Part model, mm, in its own coordinate system. Round coordinates to 2 decimals unless told otherwise and drop trailing zeros. Return JSON: item names as keys, results as strings. Group by question number.
(1) Mould opens along Y. For faces 1 (the flat face through (6, -10, -113)), 2 (the cylindrical face through (-0.631, 2.003, -113.39)), 3 (the flat face through (6, 10, -113)) say: +Y half, -Y half, draft (parallel to the pull), parting line (faces both ways), or undercut.
(2) Drill centre lines: L1, parallel to Y at x = 0, z = -156; L2, parallel to Y at x = -7.25, z = -218.5. Where is each one in solid material? Low to high. Write a range as from..to.
(3) Drop flat-ended pins along their axis: pin 1 Ø2 at (x, z) = (9.5, -172) entering from +Y; pin 2 Ø0.7 at (y, z) = (-2.5, -154) entering from +X; pin 3 Ø0.5 at (x, z) = (-2.5, -84) entering from +Y; pin 4 Ø1.5 at (x, y) = (-0.5, -6) entering from +Z. Give the stop position or say it passes through.
Autodesk Inventor part; units mm, degrees
ref_plane "C1_XY" through (0, 0, 0) normal (0, 0, 1) x (1, 0, 0)
ref_plane "C1_YZ" through (0, 0, 0) normal (1, 0, 0) x (0, 1, 0)
ref_plane "C1_ZX" through (0, 0, 0) normal (0, 1, 0) x (0, 0, 1)
sketch "Sketch_75" plane through (0, 0, 0) normal (0, 0, 1) x (1, 0, 0)
  line L0 (-10, 3) -> (-8, 3)
  line L1 (-8, 3) -> (-8, 6)
  line L2 (-8, 6) -> (-7.0607, 6)
  line L3 (-7.0607, 6) -> (-4, 2.9393)
  line L4 (-4, 2.9393) -> (-4, 0.6536)
  arc A0 (-4, 0.6536) -> (-3.933, 0.4036) centre (-3.5, 0.6536) ccw
  line L5 (-3.933, 0.4036) -> (-3.7, 0)
  line L6 (-3.7, 0) -> (-3.933, -0.4036)
  arc A1 (-3.933, -0.4036) -> (-3.933, -0.9036) centre (-3.5, -0.6536) ccw
  line L7 (-3.933, -0.9036) -> (-3.751, -1.2189)
  line L8 (-3.751, -1.2189) -> (-4, -2.5)
  line L9 (-4, -2.5) -> (-4, -2.9393)
  line L10 (-4, -2.9393) -> (-7.0607, -6)
  line L11 (-7.0607, -6) -> (-8, -6)
  line L12 (-8, -6) -> (-8, -3)
  line L13 (-8, -3) -> (-10, -3)
  line L14 (-10, -3) -> (-10, -9)
  arc A2 (-10, -9) -> (-9, -10) centre (-9, -9) ccw
  line L15 (-9, -10) -> (-3, -10)
  line L16 (-3, -10) -> (-3, -8)
  line L17 (-3, -8) -> (-6, -8)
  line L18 (-6, -8) -> (-6, -7.0607)
  line L19 (-6, -7.0607) -> (-2.9393, -4)
  line L20 (-2.9393, -4) -> (-0.6536, -4)
  arc A3 (-0.6536, -4) -> (-0.4036, -3.933) centre (-0.6536, -3.5) ccw
  line L21 (-0.4036, -3.933) -> (0, -3.7)
  line L22 (0, -3.7) -> (0.4036, -3.933)
  arc A4 (0.4036, -3.933) -> (0.9036, -3.933) centre (0.6536, -3.5) ccw
  line L23 (0.9036, -3.933) -> (1.2189, -3.751)
  line L24 (1.2189, -3.751) -> (2.5, -4)
  line L25 (2.5, -4) -> (2.9393, -4)
  line L26 (2.9393, -4) -> (6, -7.0607)
  line L27 (6, -7.0607) -> (6, -8)
  line L28 (6, -8) -> (3, -8)
  line L29 (3, -8) -> (3, -10)
  line L30 (3, -10) -> (9, -10)
  arc A5 (9, -10) -> (10, -9) centre (9, -9) ccw
  line L31 (10, -9) -> (10, -3)
  line L32 (10, -3) -> (8, -3)
  line L33 (8, -3) -> (8, -6)
  line L34 (8, -6) -> (7.0607, -6)
  line L35 (7.0607, -6) -> (4, -2.9393)
  line L36 (4, -2.9393) -> (4, -0.6536)
  arc A6 (4, -0.6536) -> (3.933, -0.4036) centre (3.5, -0.6536) ccw
  line L37 (3.933, -0.4036) -> (3.7, 0)
  line L38 (3.7, 0) -> (3.933, 0.4036)
  arc A7 (3.933, 0.4036) -> (3.933, 0.9036) centre (3.5, 0.6536) ccw
  line L39 (3.933, 0.9036) -> (3.751, 1.2189)
  line L40 (3.751, 1.2189) -> (4, 2.5)
  line L41 (4, 2.5) -> (4, 2.9393)
  line L42 (4, 2.9393) -> (7.0607, 6)
  line L43 (7.0607, 6) -> (8, 6)
  line L44 (8, 6) -> (8, 3)
  line L45 (8, 3) -> (10, 3)
  line L46 (10, 3) -> (10, 9)
  arc A8 (10, 9) -> (9, 10) centre (9, 9) ccw
  line L47 (9, 10) -> (3, 10)
  line L48 (3, 10) -> (3, 8)
  line L49 (3, 8) -> (6, 8)
  line L50 (6, 8) -> (6, 7.0607)
  line L51 (6, 7.0607) -> (2.9393, 4)
  line L52 (2.9393, 4) -> (0.6536, 4)
  arc A9 (0.6536, 4) -> (0.4036, 3.933) centre (0.6536, 3.5) ccw
  line L53 (0.4036, 3.933) -> (0, 3.7)
  line L54 (0, 3.7) -> (-0.4036, 3.933)
  arc A10 (-0.4036, 3.933) -> (-0.9036, 3.933) centre (-0.6536, 3.5) ccw
  line L55 (-0.9036, 3.933) -> (-1.2189, 3.751)
  line L56 (-1.2189, 3.751) -> (-2.5, 4)
  line L57 (-2.5, 4) -> (-2.9393, 4)
  line L58 (-2.9393, 4) -> (-6, 7.0607)
  line L59 (-6, 7.0607) -> (-6, 8)
  line L60 (-6, 8) -> (-3, 8)
  line L61 (-3, 8) -> (-3, 10)
  line L62 (-3, 10) -> (-9, 10)
  arc A11 (-9, 10) -> (-10, 9) centre (-9, 9) ccw
  line L63 (-10, 9) -> (-10, 3)
extrude "Extrusion1" add sketch "Sketch_75" against normal blind 230
sketch "Sketch2" plane through (0, 0, -230) normal (0, 0, -1) x (-1, 0, 0)
  point P0 (0, 0)
hole "Hole1" at (0, 0, -230) direction (0, 0, 1) diameter 4.2 depth 230
ref_plane "C1_XY" through (0, 0, 0) normal (0, 0, 1) x (1, 0, 0)
ref_plane "C1_YZ" through (0, 0, 0) normal (1, 0, 0) x (0, 1, 0)
ref_plane "C1_ZX" through (0, 0, 0) normal (0, 1, 0) x (0, 0, 1)
properties part number "NFS5-2020-230"
Computed values:
{
 "1": {"face 1": "-Y half", "face 2": "undercut", "face 3": "+Y half"},
 "2": {"L1": "-3.7..-2.1, 2.1..3.7", "L2": "-10..-6, 6..10"},
 "3": {"pin 1": "y = 10", "pin 2": "x = 4", "pin 3": "y = 4", "pin 4": "through"}
}
